The model under review builds one solid part; all positions refer to its coordinate system, in mm. Coordinates: 2 decimals unless noted, no trailing zeros. Write each loop counter-clockwise with the first axis right and the second up, starting at its lowest first coordinate (ties: lowest second). Pieces come first, ordered by that corner, then holes.
1) Add section C-C, the plane y = 91. State the section outline as (x, z) points (3 decimals), then the cut area to 3 significant figures.
2) Add section B-B, the plane x = -7. State the section outline as (y, z) points (3 decimals), then the cut area to 3 significant figures.
3) For P1, Ø1.6, axis at y = 239.5, z = 1, coming from the +X side; P2, Ø1.6, axis at x = 5.5, z = 1.5, coming from the +Y side; P3, Ø4, axis at x = 29, y = 97.5, coming from the -Z side, all flat-tipped, find the tip position at first contact; note any pin that passes through.
4) Add section D-D, the plane x = 78.5. State the section outline as (y, z) points (3 decimals).
5) Add section A-A, the plane z = 1.75. State the section outline as (x, y) points.
6) For line 1 (Y direction, x = 4.5, z = 1.7); line 2 (Y direction, x = -5, z = 1.95); line 3 (X direction, y = 38, z = 0.35), list the stretches that pass through material, from the lowest coordinate up.
from build123d import *

# Parameters (mm, degrees)
BOSS_EXTRUDE1_DEPTH = 3.175
CUT_EXTRUDE1_REACH  = 5.175
SKETCH2_W           = 29.718
SKETCH2_H           = 29.718
FILLET1_R           = 2.54


with BuildPart() as part:
    # Sketch1 → Boss-Extrude1 (new body)
    with BuildSketch(Plane.XY):
        with BuildLine():
            Line((-158.711897248, -0.694588462), (158.711897248, -0.694588462))
            ThreePointArc((158.711897248, -0.694588462), (154.323359707, 107.497469491), (118.128585461, 209.55))
            ThreePointArc((118.128585461, 209.55), (0, 280.345753402), (-118.128585461, 209.55))
            ThreePointArc((-118.128585461, 209.55), (-154.323359707, 107.497469491), (-158.711897248, -0.694588462))
        make_face()
    extrude(amount=BOSS_EXTRUDE1_DEPTH)

    # Sketch2 → Cut-Extrude1 (cut, up to next)
    with BuildSketch(Plane.XY.offset(3.175), mode=Mode.PRIVATE) as cut_extrude1_sk1:
        with Locations((0, 242.002411538)):
            Rectangle(SKETCH2_W, SKETCH2_H)
    cut_extrude1_tool1 = extrude(cut_extrude1_sk1.sketch, amount=-CUT_EXTRUDE1_REACH, mode=Mode.PRIVATE) & part.part
    add(cut_extrude1_tool1.solids().sort_by_distance((0, 242.002412, 3.175))[0], mode=Mode.SUBTRACT)

    # Fillet1
    fillet1_edges = [part.edges().sort_by_distance(p)[0] for p in [
        (14.859, 256.861411538, 1.5875),
        (14.859, 227.143411538, 1.5875),
        (-14.859, 227.143411538, 1.5875),
        (-14.859, 256.861411538, 1.5875),
    ]]
    fillet(fillet1_edges, radius=FILLET1_R)


solid = part.part
Geometry results:
1. outline: (-157.114, 0) - (157.114, 0) - (157.114, 3.175) - (-157.114, 3.175) - close
1. area: 998 mm2
2. outline: (-0.695, 0) - (227.143, 0) - (227.143, 3.175) - (-0.695, 3.175) - close; (256.861, 0) - (280.163, 0) - (280.163, 3.175) - (256.861, 3.175) - close
2. area: 797 mm2
3. P1: stops at x = 97.07
3. P2: stops at y = 280.26
3. P3: stops at z = 0
4. outline: (-0.695, 0) - (254.933, 0) - (254.933, 3.175) - (-0.695, 3.175) - close
5. outline: (-158.71, -0.69) - (158.71, -0.69) arc R361.95 ccw to (118.13, 209.55) arc R133.95 ccw to (-118.13, 209.55) arc R361.95 ccw to start; hole (-14.86, 229.68) arc R2.54 ccw to (-12.32, 227.14) - (12.32, 227.14) arc R2.54 ccw to (14.86, 229.68) - (14.86, 254.32) arc R2.54 ccw to (12.32, 256.86) - (-12.32, 256.86) arc R2.54 ccw to (-14.86, 254.32) - close
6. line 1: y = -0.69 to 227.14, 256.86 to 280.27
6. line 2: y = -0.69 to 227.14, 256.86 to 280.25
6. line 3: x = -160.88 to 160.88
